Verification items for this drawing (mm, ordinates from the low corner). Round coordinates to 2 decimals unless told otherwise and drop trailing zeros. Order: outer loops, then holes, each group sorted by start corner. A loop starts at its lowest first (then second) coordinate and runs counter-clockwise, first axis right, second up. Notation, with made-up numbers: (49.25, 8) -> (73.25, 8) arc R11 ccw to (73.25, 16) -> close; hole circle Ø6 at (60.5, 30). An arc over 180 degrees is marked (long way). Return JSON: item names as keys, results as strings. Group by question number.
Item 1: Depth check by flat-ended pin: pin 1 Ø1.5 at (x, y) = (79, 2) entering from +Z; pin 2 Ø0.9 at (x, y) = (96, 2) entering from +Z; pin 3 Ø0.9 at (x, y) = (110.5, 1) entering from -Z; pin 4 Ø1.5 at (x, z) = (87.5, 65.5) entering from +Y. Enter the tip coordinate at first touch or a pass-through.
Item 2: Sectioned sample at C-C on z = 60. Record the cut outline in (x, y).
Item 3: Sectioned sample at D-D on x = 62. Record the cut outline in (y, z), plus the area to 3 significant figures.
Item 4: Scan lines: probe 1 along X at (y, z) = (1.05, 37); probe 2 along X at (y, z) = (1.4, 56); probe 3 along X at (y, z) = (1.05, 27). Record each from-to range of solid material in increasing order. Write a range as from..to.
Item 5: Sectioned sample at A-A on z = 29. Record the cut outline in (x, y).
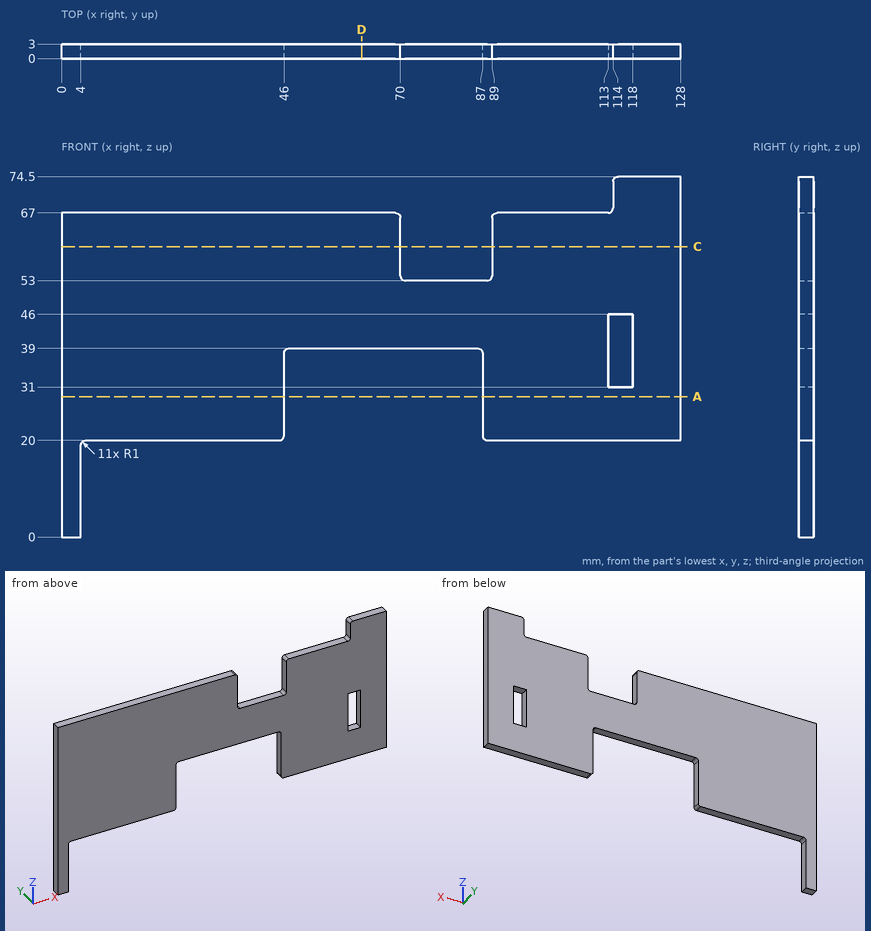
Recorded:
{
 "1": {"pin 1": "z = 53", "pin 2": "z = 67", "pin 3": "z = 20", "pin 4": "through"},
 "2": {"outline": "(0, 0) -> (70, 0) -> (70, 3) -> (0, 3) -> close; (89, 0) -> (128, 0) -> (128, 3) -> (89, 3) -> close"},
 "3": {"outline": "(0, 39) -> (3, 39) -> (3, 67) -> (0, 67) -> close", "area": "84.0 mm²"},
 "4": {"probe 1": "0..46, 87..113, 118..128", "probe 2": "0..70, 89..128", "probe 3": "0..46, 87..128"},
 "5": {"outline": "(0, 0) -> (46, 0) -> (46, 3) -> (0, 3) -> close; (87, 0) -> (128, 0) -> (128, 3) -> (87, 3) -> close"}
}
